Read the model definition and answer for the solid it produces. Units are mm, in the model's axes. A direction names the side the tool comes from. Give positions to 0.01 mm unless a question says otherwise; leave off trailing zeros. Write each loop counter-clockwise with the first axis right and the second up, starting at its lowest first coordinate (ties: lowest second). Pieces come first, ordered by that corner, then holes. Notation, with made-up numbers: (25.5, -38.5) -> (78.5, -38.5) arc R24 ccw to (78.5, -26.5) -> close; hole circle Ø7 at (62, -25.75). An arc over 180 degrees is marked (long way). Use a Markdown table: item, result.
from build123d import *

# Parameters (mm, degrees)
BOSS_EXTRUDE1_DEPTH  = 2
SKETCH2_W            = 5
SKETCH2_H            = 25
SKETCH2_W_2          = 20
BOSS_EXTRUDE2_DEPTH  = 20
SKETCH3_W            = 25
SKETCH3_H            = 2
BOSS_EXTRUDE3_DEPTH  = 25
SKETCH4_W            = 25
SKETCH4_H            = 25
BOSS_EXTRUDE4_DEPTH  = 7
BOSS_EXTRUDE5_DEPTH  = 5
SKETCH6_W            = 50
SKETCH6_H            = 25
BOSS_EXTRUDE6_DEPTH  = 5
BOSS_EXTRUDE7_DEPTH  = 30
CUT_EXTRUDE2_DEPTH   = 30
SKETCH10_W           = 5
SKETCH10_H           = 25
CUT_EXTRUDE3_DEPTH   = 20
SKETCH11_W           = 25
SKETCH11_H           = 25
CUT_EXTRUDE4_DEPTH   = 7
SKETCH13_W           = 5
SKETCH13_H           = 25
CUT_EXTRUDE5_DEPTH   = 10
BOSS_EXTRUDE8_REACH  = 12
SKETCH14_W           = 10
SKETCH14_H           = 5
SKETCH15_W           = 2.5
SKETCH15_H           = 25
CUT_EXTRUDE6_DEPTH   = 15
SKETCH16_W           = 5
SKETCH16_H           = 15
CUT_EXTRUDE7_DEPTH   = 26
SKETCH17_W           = 5
SKETCH17_H           = 15
CUT_EXTRUDE8_DEPTH   = 43.5
SKETCH18_W           = 5
SKETCH18_H           = 15
CUT_EXTRUDE9_DEPTH   = 6
CUT_EXTRUDE10_DEPTH  = 43.5
CUT_EXTRUDE11_DEPTH  = 43.5
SKETCH21_W           = 5
SKETCH21_H           = 5
SKETCH21_H_2         = 15
BOSS_EXTRUDE9_DEPTH  = 5
SKETCH22_W           = 5
SKETCH22_H           = 5
SKETCH22_W_2         = 50
SKETCH22_H_2         = 15
CUT_EXTRUDE12_DEPTH  = 6
SKETCH23_W           = 5
SKETCH23_H           = 5
CUT_EXTRUDE13_DEPTH  = 6
BOSS_EXTRUDE10_DEPTH = 15
BOSS_EXTRUDE11_DEPTH = 5
SKETCH26_W           = 65
SKETCH26_H           = 5
CUT_EXTRUDE14_DEPTH  = 20


with BuildPart() as part:
    # Sketch1 → Boss-Extrude1 (new body)
    with BuildSketch(Plane.XY):
        Polygon((-5, 75), (2.5, 25), (2.5, 0), (22.5, 0), (22.5, 25), (30, 75), (30, 100), (25, 100), (25, 75), (0, 75), (0, 100), (-5, 100), align=None)
    extrude(amount=BOSS_EXTRUDE1_DEPTH)

    # Sketch2 → Boss-Extrude2 (add)
    with BuildSketch(Plane(origin=(0, 0, 0), x_dir=(-1, 0, 0), z_dir=(0, 0, -1))):
        with Locations((-27.5, 87.5)):
            Rectangle(SKETCH2_W, SKETCH2_H)
        with Locations((2.5, 87.5)):
            Rectangle(SKETCH2_W, SKETCH2_H)
        with Locations((-12.5, 12.5)):
            Rectangle(SKETCH2_W_2, SKETCH2_H)
    extrude(amount=BOSS_EXTRUDE2_DEPTH)

    # Sketch3 → Boss-Extrude3 (add)
    with BuildSketch(Plane(origin=(0, 75, 0), x_dir=(1, 0, 0), z_dir=(0, 1, 0))):
        with Locations((12.5, -1)):
            Rectangle(SKETCH3_W, SKETCH3_H)
    extrude(amount=BOSS_EXTRUDE3_DEPTH)

    # Sketch4 → Boss-Extrude4 (add)
    with BuildSketch(Plane(origin=(0, 0, 0), x_dir=(-1, 0, 0), z_dir=(0, 0, -1))):
        with Locations((-12.5, 87.5)):
            Rectangle(SKETCH4_W, SKETCH4_H)
    extrude(amount=BOSS_EXTRUDE4_DEPTH)

    # Sketch5 → Boss-Extrude5 (add)
    with BuildSketch(Plane(origin=(0, 0, 0), x_dir=(-1, 0, 0), z_dir=(0, 0, -1))):
        Polygon((5, 75), (5, 0), (-2.5, 0), (-22.5, 0), (-30, 0), (-30, 75), (-30, 100), (5, 100), align=None)
    extrude(amount=-BOSS_EXTRUDE5_DEPTH)

    # Sketch6 → Boss-Extrude6 (add)
    with BuildSketch(Plane.XY.offset(5)):
        with Locations((12.5, 12.5)):
            Rectangle(SKETCH6_W, SKETCH6_H)
    extrude(amount=-BOSS_EXTRUDE6_DEPTH)

    # Sketch8 → Boss-Extrude7 (add)
    with BuildSketch(Plane.XZ.offset(-75)):
        Polygon((-5, 0), (-5, -20), (0, -20), (0, -7), (25, -7), (25, -20), (30, -20), (30, 0), align=None)
    extrude(amount=BOSS_EXTRUDE7_DEPTH)

    # Sketch9 → Cut-Extrude2 (cut)
    with BuildSketch(Plane(origin=(0, 100, 0), x_dir=(1, 0, 0), z_dir=(0, 1, 0))):
        Polygon((30, 20), (25, 20), (25, 7), (0, 7), (0, 20), (-5, 20), (-5, -5), (30, -5), align=None)
    extrude(amount=-CUT_EXTRUDE2_DEPTH, mode=Mode.SUBTRACT)

    # Sketch10 → Cut-Extrude3 (cut)
    with BuildSketch(Plane(origin=(0, 0, -20), x_dir=(-1, 0, 0), z_dir=(0, 0, -1))):
        with Locations((-20, 12.5)):
            Rectangle(SKETCH10_W, SKETCH10_H)
        with Locations((-5, 12.5)):
            Rectangle(SKETCH10_W, SKETCH10_H)
    extrude(amount=-CUT_EXTRUDE3_DEPTH, mode=Mode.SUBTRACT)

    # Sketch11 → Cut-Extrude4 (cut)
    with BuildSketch(Plane(origin=(0, 0, -7), x_dir=(-1, 0, 0), z_dir=(0, 0, -1))):
        with Locations((-12.5, 57.5)):
            Rectangle(SKETCH11_W, SKETCH11_H)
    extrude(amount=-CUT_EXTRUDE4_DEPTH, mode=Mode.SUBTRACT)

    # Sketch13 → Cut-Extrude5 (cut)
    with BuildSketch(Plane(origin=(17.5, 0, 0), x_dir=(0, 0, -1), z_dir=(1, 0, 0))):
        Polygon((5, 25), (5, 20), (10, 20), (10, 5), (0, 5), (0, 25), align=None)
        with Locations((17.5, 12.5)):
            Rectangle(SKETCH13_W, SKETCH13_H)
    extrude(amount=-CUT_EXTRUDE5_DEPTH, mode=Mode.SUBTRACT)

    # Sketch14 → Boss-Extrude8 (add, up to next)
    with BuildSketch(Plane.XY.offset(-5), mode=Mode.PRIVATE) as boss_extrude8_sk1:
        with Locations((12.5, 22.5)):
            Rectangle(SKETCH14_W, SKETCH14_H)
    boss_extrude8_tool1 = extrude(boss_extrude8_sk1.sketch, amount=BOSS_EXTRUDE8_REACH, mode=Mode.PRIVATE) - part.part
    add(boss_extrude8_tool1.solids().sort_by_distance((12.5, 22.5, -5))[0])

    # Sketch15 → Cut-Extrude6 (cut)
    with BuildSketch(Plane(origin=(0, 0, -15), x_dir=(-1, 0, 0), z_dir=(0, 0, -1))):
        with Locations((-8.75, 12.5)):
            Rectangle(SKETCH15_W, SKETCH15_H)
        with Locations((-16.25, 12.5)):
            Rectangle(SKETCH15_W, SKETCH15_H)
    extrude(amount=-CUT_EXTRUDE6_DEPTH, mode=Mode.SUBTRACT)

    # Sketch16 → Cut-Extrude7 (cut, through all)
    with BuildSketch(Plane.XY.offset(5)):
        with Locations((-5, 12.5)):
            Rectangle(SKETCH16_W, SKETCH16_H)
        with Locations((30, 12.5)):
            Rectangle(SKETCH16_W, SKETCH16_H)
    extrude(amount=-CUT_EXTRUDE7_DEPTH, mode=Mode.SUBTRACT)

    # Sketch17 → Cut-Extrude8 (cut, through all)
    with BuildSketch(Plane(origin=(30, 0, 0), x_dir=(0, 0, -1), z_dir=(1, 0, 0))):
        with Locations((2.5, 57.5)):
            Rectangle(SKETCH17_W, SKETCH17_H)
    extrude(amount=-CUT_EXTRUDE8_DEPTH, mode=Mode.SUBTRACT)

    # Sketch18 → Cut-Extrude9 (cut, through all)
    with BuildSketch(Plane(origin=(0, 0, 0), x_dir=(-1, 0, 0), z_dir=(0, 0, -1))):
        with Locations((-2.5, 57.5)):
            Rectangle(SKETCH18_W, SKETCH18_H)
        with Locations((-22.5, 57.5)):
            Rectangle(SKETCH18_W, SKETCH18_H)
    extrude(amount=-CUT_EXTRUDE9_DEPTH, mode=Mode.SUBTRACT)

    # Sketch19 → Cut-Extrude10 (cut, through all)
    with BuildSketch(Plane(origin=(30, 0, 0), x_dir=(0, 0, -1), z_dir=(1, 0, 0))):
        Polygon((5, 60), (10, 60), (10, 45), (20, 45), (20, 70), (-5, 70), (-5, 60), (0, 60), align=None)
    extrude(amount=-CUT_EXTRUDE10_DEPTH, mode=Mode.SUBTRACT)

    # Sketch20 → Cut-Extrude11 (cut, through all)
    with BuildSketch(Plane(origin=(30, 0, 0), x_dir=(0, 0, -1), z_dir=(1, 0, 0))):
        Polygon((10, 45), (15, 25), (15, 0), (0, 0), (0, 60), (10, 60), align=None)
    extrude(amount=-CUT_EXTRUDE11_DEPTH, mode=Mode.SUBTRACT)

    # Sketch21 → Boss-Extrude9 (add)
    with BuildSketch(Plane(origin=(0, 0, 0), x_dir=(-1, 0, 0), z_dir=(0, 0, -1))):
        with Locations((-2.5, 57.5)):
            Rectangle(SKETCH21_W, SKETCH21_H)
        with Locations((-22.5, 57.5)):
            Rectangle(SKETCH21_W, SKETCH21_H)
        with Locations((5, 12.5)):
            Rectangle(SKETCH21_W, SKETCH21_H_2)
        with Locations((-30, 12.5)):
            Rectangle(SKETCH21_W, SKETCH21_H_2)
    extrude(amount=-BOSS_EXTRUDE9_DEPTH)

    # Sketch22 → Cut-Extrude12 (cut, through all)
    with BuildSketch(Plane(origin=(0, 0, 0), x_dir=(-1, 0, 0), z_dir=(0, 0, -1))):
        with Locations((-12.5, 22.5)):
            Rectangle(SKETCH22_W, SKETCH22_H)
        with Locations((-12.5, 7.5)):
            Rectangle(SKETCH22_W_2, SKETCH22_H_2)
    extrude(amount=-CUT_EXTRUDE12_DEPTH, mode=Mode.SUBTRACT)

    # Sketch23 → Cut-Extrude13 (cut, through all)
    with BuildSketch(Plane(origin=(0, 0, 0), x_dir=(-1, 0, 0), z_dir=(0, 0, -1))):
        with Locations((-22.5, 32.5)):
            Rectangle(SKETCH23_W, SKETCH23_H)
        with Locations((-2.5, 32.5)):
            Rectangle(SKETCH23_W, SKETCH23_H)
    extrude(amount=-CUT_EXTRUDE13_DEPTH, mode=Mode.SUBTRACT)

    # Sketch24 → Boss-Extrude10 (add)
    with BuildSketch(Plane.XZ.offset(-25)):
        Polygon((-12.5, 5), (-20, 5), (-20, 0), (-12.5, 0), (37.5, 0), (45, 0), (45, 5), (37.5, 5), align=None)
    extrude(amount=BOSS_EXTRUDE10_DEPTH)

    # Sketch25 → Boss-Extrude11 (add, through all)
    with BuildSketch(Plane.XY.offset(5)):
        Polygon((45, 25), (30, 25), (30, 60), align=None)
        Polygon((-5, 25), (-5, 60), (-20, 25), align=None)
    extrude(amount=-BOSS_EXTRUDE11_DEPTH)

    # Sketch26 → Cut-Extrude14 (cut)
    with BuildSketch(Plane(origin=(0, 60, 0), x_dir=(1, 0, 0), z_dir=(0, 1, 0))):
        with Locations((12.5, -2.5)):
            Rectangle(SKETCH26_W, SKETCH26_H)
    extrude(amount=-CUT_EXTRUDE14_DEPTH, mode=Mode.SUBTRACT)


solid = part.part
Item 1: For a pull along X with two mould halves and no side action, classify faces 1 (the face through (13, 25, 0)), 2 (the face through (-16.741, 32.605, 2.535)), 3 (the face through (0, 32, 2)) as +X half, -X half, draft (parallel to the pull), parting line (faces both ways), or undercut.
Return value:
| item | result |
|---|---|
| face 1 | draft |
| face 2 | -X half |
| face 3 | undercut |
Item 2: A tool of negligible diameter and unlimited length cuts with its end or side. For faces 4 (the face through (20, 32, 2)), 5 (the face through (-20, 18, 3)), from which of +Z, -Z, +X, -X, +Y, -Y can it reach the whole face along a straight path? Write none if from no direction.
Return value:
| item | result |
|---|---|
| face 4 | +Z, -Z |
| face 5 | +Z, -Z, -X, +Y, -Y |
Item 3: Straight lines are drawn through the part: line 1 along X through (y, z) = (34, 4.85); line 2 along Y through (x, z) = (4, 3.45); line 3 along X through (y, z) = (28, 4.3). For each, find the intervals that lie inside material, in ascending order. Write a range as [from, to].
Return value:
| item | result |
|---|---|
| line 1 | [-16.14, 0], [5, 20], [25, 41.14] |
| line 2 | [10, 30], [35, 40] |
| line 3 | [-18.71, 43.71] |
Item 4: A cutting plane is placed at D-D (y = 37.75). Give the vertices of the cut face in (x, z).
Return value:
| item | result |
|---|---|
| outline | (-14.54, 0) -> (39.54, 0) -> (39.54, 5) -> (-14.54, 5) -> close |
Item 5: A cutting plane is placed at A-A (x = 1.5). Give the vertices of the cut face in (y, z).
Return value:
| item | result |
|---|---|
| outline | (10, 0) -> (30, 0) -> (30, 5) -> (10, 5) -> close; (35, 0) -> (40, 0) -> (40, 5) -> (35, 5) -> close |
Item 6: This flat-tipped pin is pushed along its axis until it touches: P1, Ø2.5, axis at y = 31.5, z = 2, coming from the -X side. Where does it stop, or does it pass through?
Return value:
| item | result |
|---|---|
| P1 | x = -17.75 |
Item 7: A cutting plane is placed at B-B (z = 4.15). Give the vertices of the cut face in (x, y), then the cut area to 3 significant figures.
Return value:
| item | result |
|---|---|
| outline | (-20, 10) -> (45, 10) -> (45, 25) -> (38.57, 40) -> (-13.57, 40) -> (-20, 25) -> close; hole (0, 30) -> (5, 30) -> (5, 35) -> (0, 35) -> close; hole (20, 30) -> (25, 30) -> (25, 35) -> (20, 35) -> close |
| area | 1,800 mm^2 |
Item 8: A cutting plane is placed at C-C (y = 34.25). Give the vertices of the cut face in (x, z).
Return value:
| item | result |
|---|---|
| outline | (-16.04, 0) -> (0, 0) -> (0, 5) -> (-16.04, 5) -> close; (5, 0) -> (20, 0) -> (20, 5) -> (5, 5) -> close; (25, 0) -> (41.04, 0) -> (41.04, 5) -> (25, 5) -> close |
